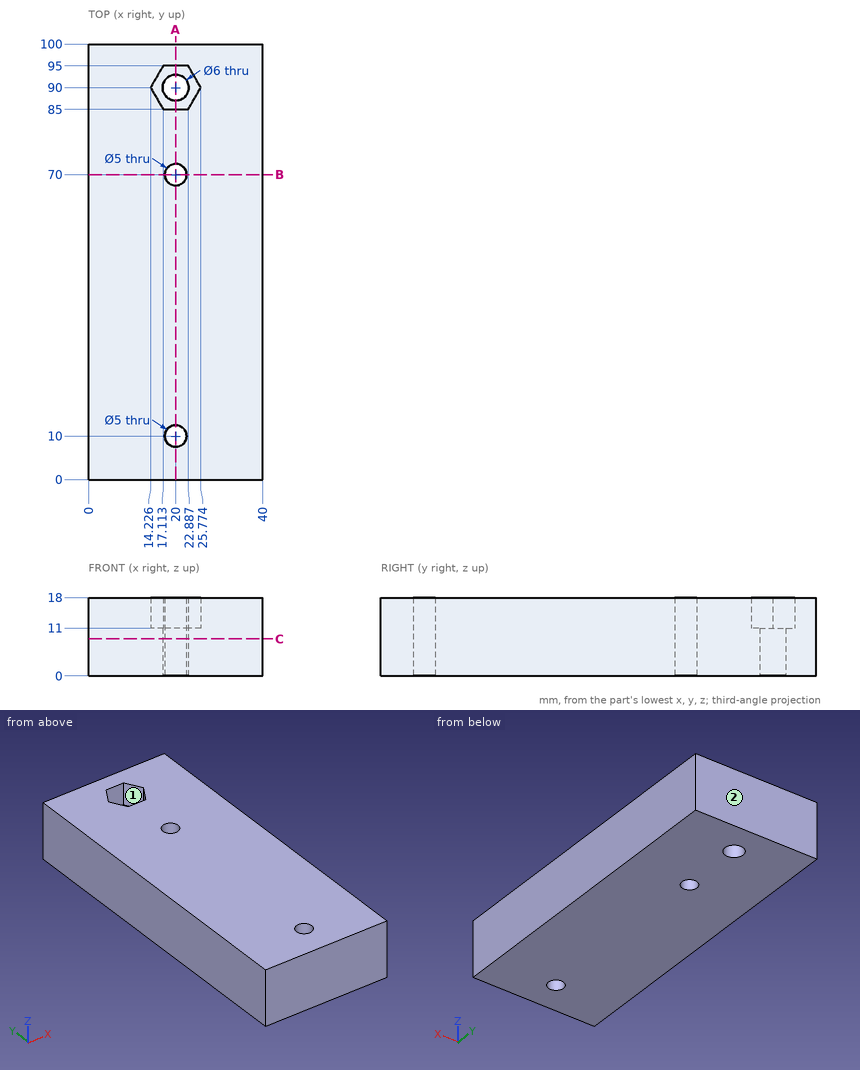
Design review of the part shown in the three views and the two pictorial views. Dimensions are in mm from the part's minimum x, y and z. A direction names the side the tool comes from. Coordinates: 2 decimals unless noted, no trailing zeros. Write each loop counter-clockwise with the first axis right and the second up, starting at its lowest first coordinate (ties: lowest second). Pieces come first, ordered by that corner, then holes.
(1) Add section C-C on z = 8.5. Give the boundary of the cut face in (x, y), then the cut area to 3 significant figures.
(2) Add section A-A on x = 20. Give the boundary of the cut face in (y, z).
(3) Wall thickness on probe 1 along Y at (x, z) = (20, 10); probe 2 along X at (y, z) = (10, 5.75); probe 3 along Y at (x, z) = (18.5, 10.25): over which ranges is each line inside the solid? List them lowest first.
(4) Add section B-B on y = 70. Give the boundary of the cut face in (x, z).
(5) For pin 1 Ø6.5 at (x, y) = (20, 10) entering from -Z; pin 2 Ø5 at (x, y) = (19, 88.5) entering from +Z, all flat-tipped, find the tip position at first contact; note any pin that passes through.
(6) Tool access review of the marked faces 1 and 2: name each direction out of +Z, -Z, +X, -X, +Y, -Y from which nothing blocks a thin tool from reaching the whole face with its end or side.
Answer sheet:
1. outline: (0, 0) - (40, 0) - (40, 100) - (0, 100) - close; hole circle Ø6 at (20, 90); hole circle Ø5 at (20, 10); hole circle Ø5 at (20, 70)
1. area: 3,930 mm2
2. outline: (0, 0) - (7.5, 0) - (7.5, 18) - (0, 18) - close; (12.5, 0) - (67.5, 0) - (67.5, 18) - (12.5, 18) - close; (72.5, 0) - (87, 0) - (87, 11) - (85, 11) - (85, 18) - (72.5, 18) - close; (93, 0) - (100, 0) - (100, 18) - (95, 18) - (95, 11) - (93, 11) - close
3. probe 1: y = 0 to 7.5, 12.5 to 67.5, 72.5 to 87, 93 to 100
3. probe 2: x = 0 to 17.5, 22.5 to 40
3. probe 3: y = 0 to 8, 12 to 68, 72 to 87.4, 92.6 to 100
4. outline: (0, 0) - (17.5, 0) - (17.5, 18) - (0, 18) - close; (22.5, 0) - (40, 0) - (40, 18) - (22.5, 18) - close
5. pin 1: stops at z = 0
5. pin 2: stops at z = 11
6. face 1: +Z
6. face 2: +Z, -Z, +X, -X, +Y
